from build123d import *

# Parameters (mm, degrees)
SKETCH1_R               = 4
SKETCH1_R_2             = 1
BOSS_EXTRUDE1_DEPTH     = 1
BOSS_EXTRUDE2_DEPTH     = 4
BOSS_EXTRUDE3_DEPTH     = 3
SKETCH6_W               = 5
SKETCH6_H               = 3
CUT_EXTRUDE1_DEPTH      = 6
SKETCH7_R               = 4
CUT_EXTRUDE2_DEPTH      = 3
CUT_EXTRUDE2_DEPTH_BACK = 1
BOSS_EXTRUDE4_DEPTH     = 2


with BuildPart() as part:
    # Sketch1 → Boss-Extrude1 (new body)
    with BuildSketch(Plane(origin=(0, 0, 0), x_dir=(1, 0, 0), z_dir=(0, 1, 0))):
        Circle(SKETCH1_R)
        Circle(SKETCH1_R_2, mode=Mode.SUBTRACT)
        with BuildLine():
            ThreePointArc((0, -5), (5, 0), (0, 5))
            Line((0, 5), (0, 4))
            ThreePointArc((0, 4), (2.828427125, 2.828427125), (4, 0))
            ThreePointArc((4, 0), (2.828427125, -2.828427125), (0, -4))
            Line((0, -4), (0, -5))
        make_face()
        with BuildLine():
            Line((0, 4), (0, 5))
            ThreePointArc((0, 5), (-3.535533906, 3.535533906), (-5, 0))
            Line((-5, 0), (-4, 0))
            ThreePointArc((-4, 0), (-2.828427125, 2.828427125), (0, 4))
        make_face()
    extrude(amount=BOSS_EXTRUDE1_DEPTH)

    # Sketch2 → Boss-Extrude2 (add)
    with BuildSketch(Plane(origin=(0, 1, 0), x_dir=(1, 0, 0), z_dir=(0, 1, 0))):
        with BuildLine():
            Line((0, 3), (0, 5))
            ThreePointArc((0, 5), (5, 0), (0, -5))
            Line((0, -5), (0, -3))
            ThreePointArc((0, -3), (3, 0), (0, 3))
        make_face()
    extrude(amount=BOSS_EXTRUDE2_DEPTH)

    # Sketch4 → Boss-Extrude3 (add)
    with BuildSketch(Plane(origin=(0, 5, 0), x_dir=(1, 0, 0), z_dir=(0, 1, 0))):
        with BuildLine():
            Line((0, 5), (0, 4))
            ThreePointArc((0, 4), (3.883896034, 0), (0, -4))
            Line((0, -4), (0, -5))
            ThreePointArc((0, -5), (5, 0), (0, 5))
        make_face()
    extrude(amount=BOSS_EXTRUDE3_DEPTH)

    # Sketch6 → Cut-Extrude1 (cut)
    with BuildSketch(Plane.ZY):
        with Locations((2.5, 6.5)):
            Rectangle(SKETCH6_W, SKETCH6_H)
    extrude(amount=-CUT_EXTRUDE1_DEPTH, mode=Mode.SUBTRACT)

    # Sketch7 → Cut-Extrude2 (cut, two sides)
    with BuildSketch(Plane(origin=(0, 5, 0), x_dir=(1, 0, 0), z_dir=(0, 1, 0))) as cut_extrude2_sk:
        Circle(SKETCH7_R)
    extrude(amount=CUT_EXTRUDE2_DEPTH, mode=Mode.SUBTRACT)
    extrude(cut_extrude2_sk.sketch, amount=-CUT_EXTRUDE2_DEPTH_BACK, mode=Mode.SUBTRACT)

    # Sketch8 → Boss-Extrude4 (add)
    with BuildSketch(Plane(origin=(0, 1, 0), x_dir=(1, 0, 0), z_dir=(0, 1, 0))):
        with BuildLine():
            Line((0, 5), (0, 4))
            ThreePointArc((0, 4), (-2.828427125, 2.828427125), (-4, 0))
            Line((-4, 0), (-5, 0))
            ThreePointArc((-5, 0), (-3.535533906, 3.535533906), (0, 5))
        make_face()
    extrude(amount=BOSS_EXTRUDE4_DEPTH)


solid = part.part
The model under review builds one solid part; all positions refer to its coordinate system, in mm. A direction names the side the tool comes from. Give positions to 0.01 mm unless a question says otherwise; leave off trailing zeros. Write each loop counter-clockwise with the first axis right and the second up, starting at its lowest first coordinate (ties: lowest second). Pieces come first, ordered by that corner, then holes.
1. Wall thickness on L1, parallel to Y at x = 2, z = 4.25; L2, parallel to Y at x = 1, z = 0.25; L3, parallel to Z at x = 0.5, y = 1.75: over which ranges is each line inside the solid? List them lowest first.
2. Tool access review of faces 4 (the cylindrical face through (-2.797, 1.986, -2.859)), 5 (the flat face through (0, 2, 4)), 6 (the cylindrical face through (3.12, 5.58, -2.5)), 7 (the cylindrical face through (3, 2, 0)): name each direction out of +Z, -Z, +X, -X, +Y, -Y from which nothing blocks a thin tool from reaching the whole face with its end or side.
3. For P1, Ø2.5, axis at x = 2, z = 3.5, coming from the +Y side; P2, Ø1, axis at x = -2.5, z = 2, coming from the +Y side; P3, Ø0.5, axis at x = -4.5, y = 1.5, coming from the +Z side; P4, Ø1.6, axis at x = 0, z = 0, coming from the -Y side, all flat-tipped, find the tip position at first contact; note any pin that passes through.
4. Add section B-B, the plane x = 2. Write out the cut boundary in (y, z), plus the area to 3 significant figures.
5. Add section D-D, the plane x = -2.5. Write out the cut boundary in (y, z).
6. Add section A-A, the plane y = 2.5. Write out the cut boundary in (x, z), plus the area to 3 significant figures.
7. Add section C-C, the plane z = -2. Write out the cut boundary in (x, y), plus the area to 3 significant figures.
8. Draft analysis for pull direction X (two halves, no side actions). For faces 1 (the cylindrical face through (-2.859, 0.493, 2.797)), 2 (the flat face through (3, 8, -3)), 3 (the flat face through (-1.3, 1, -0.1)), state which applies: +X half, -X half, draft (parallel to the pull), parting line (faces both ways), or undercut.
Worked answers:
1. L1: y = 0 to 5
1. L2: y = 0 to 1
1. L3: z = -4.97 to -2.96, 2.96 to 4.97
2. face 4: +Z, +Y
2. face 5: +Z, -X, +Y
2. face 6: -X, +Y
2. face 7: +Y
3. P1: stops at y = 5
3. P2: stops at y = 1
3. P3: stops at z = 0
3. P4: passes through
4. outline: (0, -4.58) - (8, -4.58) - (8, -3.46) - (4, -3.46) - (4, -2.24) - (1, -2.24) - (1, 2.24) - (4, 2.24) - (4, 3.46) - (5, 3.46) - (5, 4.58) - (0, 4.58) - close
4. area: 28.8 mm2
5. outline: (0, -4.33) - (3, -4.33) - (3, -3.12) - (1, -3.12) - (1, 3.12) - (0, 3.12) - close
6. outline: (-5, 0) arc R5 ccw (long way) to (0, 5) - (0, 3) arc R3 cw to (0, -3) - (0, -4) arc R4 cw to (-4, 0) - close
6. area: 32.2 mm2
7. outline: (-4.58, 0) - (4.58, 0) - (4.58, 8) - (3.46, 8) - (3.46, 4) - (2.24, 4) - (2.24, 1) - (-3.46, 1) - (-3.46, 3) - (-4.58, 3) - close
7. area: 22.9 mm2
8. face 1: -X half
8. face 2: draft
8. face 3: undercut
